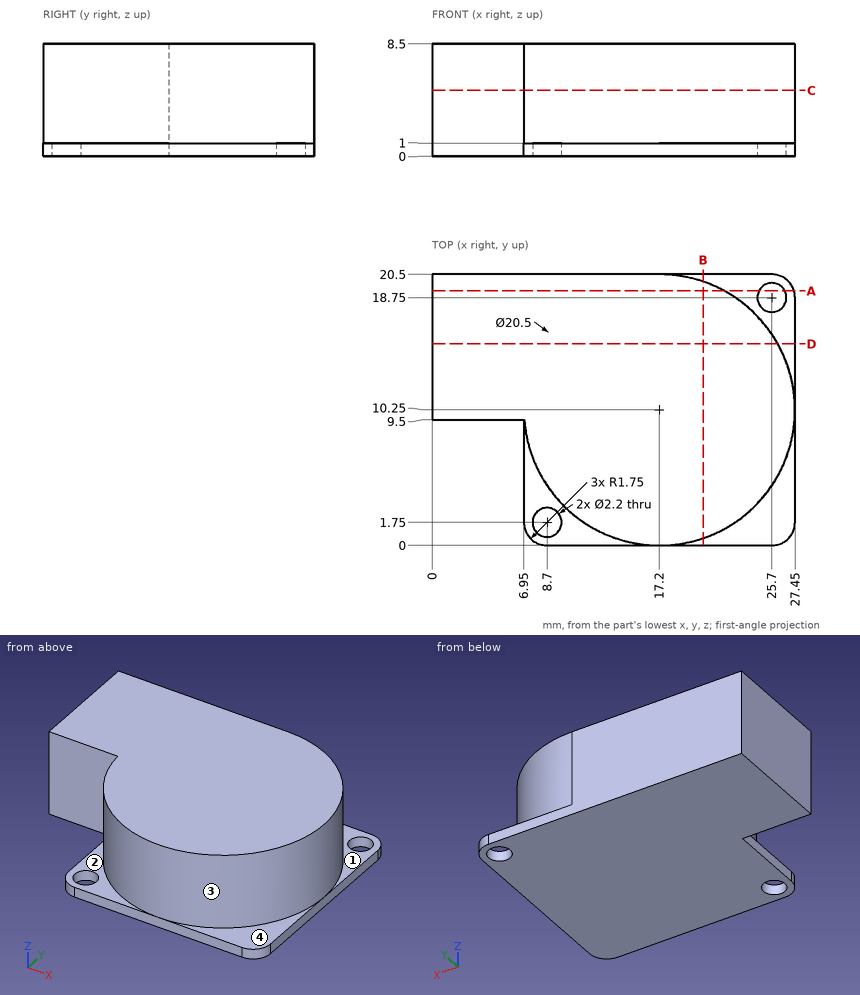
Design review of the part shown in the three views and the two pictorial views. Dimensions are in mm from the part's minimum x, y and z. A direction names the side the tool comes from. Round coordinates to 2 decimals unless told otherwise and drop trailing zeros. Write each loop counter-clockwise with the first axis right and the second up, starting at its lowest first coordinate (ties: lowest second). Pieces come first, ordered by that corner, then holes. Notation, with made-up numbers: (7, 47.5) -> (41, 47.5) arc R21 cw to (41, 55.5) -> close; hole circle Ø1 at (28, 46.25). An arc over 180 degrees is marked (long way). Answer as a JSON object with one key per item and string values.
1. We need section C-C on z = 5. State the section outline as (x, y) points.
Results found:
{"outline": "(0, 9.5) -> (6.98, 9.5) arc R10.25 ccw (long way) to (17.2, 20.5) -> (0, 20.5) -> close"}
2. We need section D-D on y = 15.25. State the section outline as (x, z) points.
Results found:
{"outline": "(0, 0) -> (27.45, 0) -> (27.45, 1) -> (26.15, 1) -> (26.15, 8.5) -> (0, 8.5) -> close"}
3. Clearance check with flat-ended pins moving along their axes: pin 1 (1 mm diameter, centred on x = 8, z = 4, fed in from -Y); pin 2 (4 mm diameter, centred on y = 14.5, z = 3.5, fed in from +X); pin 3 (1.1 mm diameter, centred on y = 5.5, z = 0.5, fed in from -X); pin 4 (5 mm diameter, centred on y = 16, z = 5.5, fed in from -X). State where each tip first meets the part, or that it passes through.
Results found:
{"pin 1": "stops at y = 4.83", "pin 2": "stops at x = 27.2", "pin 3": "stops at x = 6.95", "pin 4": "stops at x = 0"}
4. Machinability: for the marked faces 1, 2, 3 and 4, which of the approach directions +Z, -Z, +X, -X, +Y, -Y give a long, thin tool a straight path to every point of the face, cutting with its end or side? Answer none if there is none.
Results found:
{"face 1": "+Z, +X, +Y", "face 2": "+Z, -X, -Y", "face 3": "+Z", "face 4": "+Z, +X, -Y"}
5. To check wall thickness, follow line 1 along Y through (x, z) = (8.7, 0.65); line 2 along Y through (x, z) = (25.7, 0.65); line 3 along Z through (x, y) = (24.25, 2). State the ranges of each line that lie inside material, in increasing order.
Results found:
{"line 1": "y = 0 to 0.65, 2.85 to 20.5", "line 2": "y = 0 to 17.65, 19.85 to 20.5", "line 3": "z = 0 to 1"}
6. We need section A-A on y = 19.25. State the section outline as (x, z) points, and give its area (3 significant figures).
Results found:
{"outline": "(0, 0) -> (24.72, 0) -> (24.72, 1) -> (22.11, 1) -> (22.11, 8.5) -> (0, 8.5) -> close; (26.68, 0) -> (27.38, 0) -> (27.38, 1) -> (26.68, 1) -> close", "area": "191 mm^2"}
7. We need section B-B on x = 20.5. State the section outline as (y, z) points, and give its area (3 significant figures).
Results found:
{"outline": "(0, 0) -> (20.5, 0) -> (20.5, 1) -> (19.95, 1) -> (19.95, 8.5) -> (0.55, 8.5) -> (0.55, 1) -> (0, 1) -> close", "area": "166 mm^2"}
